Check sheet for the modelled part. Datum: model origin and axes. Units: mm. Face numbers are marked on the shaded views. A direction names the side the tool comes from. Give positions to 0.01 mm unless a question says otherwise; leave off trailing zeros. Order: outer loops, then holes, each group sorted by start corner. A loop starts at its lowest first (then second) coordinate and runs counter-clockwise, first axis right, second up.
Item 1: Gauge pin test, flat ends, axial feed: P1, Ø2, axis at x = 3.5, y = 3.5, coming from the +Z side; P2, Ø9.5, axis at x = 0, z = 0, coming from the -Y side; P3, Ø1.2, axis at x = -4, y = 3.5, coming from the +Z side; P4, Ø1.5, axis at y = 2, z = -35.5, coming from the -X side. Record the tip position at first contact, or that the pin passes through.
Item 2: Sectioned sample at D-D on x = -10. Record the boundary of the cut face in (y, z), and give its area (3 significant figures).
Item 3: Sectioned sample at B-B on z = 0. Record the boundary of the cut face in (x, y), and give its area (3 significant figures).
Item 4: Sectioned sample at A-A on x = 0. Record the boundary of the cut face in (y, z), and give its area (4 significant figures).
Item 5: Release check for a two-part mould opening along X. For the marked faces 3 and 4 record: released by +X, released by -X, zero draft, split by the parting line, or undercut.
Item 6: Access from +Z, -Z, +X, -X, +Y, -Y to the whole of each face (thin tool, end or side, straight path). Record for the marked faces 1 and 2.
Item 7: Material ranges on line 1 along X through (y, z) = (2.15, 0); line 2 along Z through (x, y) = (-3.1, 1.9); line 3 along X through (y, z) = (4.6, 1), recorded low to high.
Item 8: Sectioned sample at C-C on y = 2.6. Record the boundary of the cut face in (x, z), and give its area (3 significant figures).
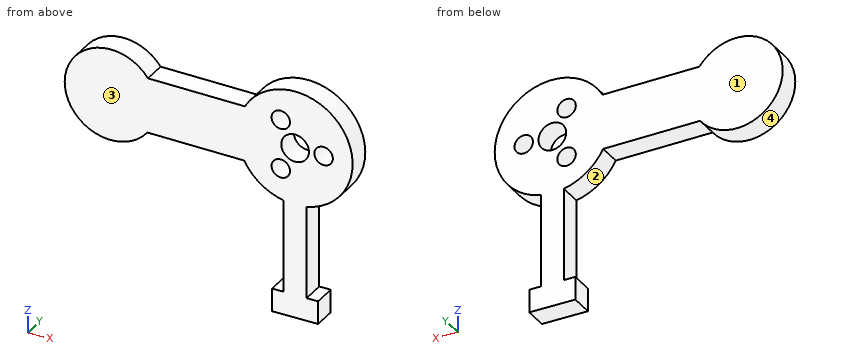
from build123d import *

# Parameters (mm, degrees)
SKETCH1_R           = 2
SKETCH1_R_2         = 3
BOSS_EXTRUDE1_DEPTH = 5


with BuildPart() as part:
    # Sketch1 → Boss-Extrude1 (new body)
    with BuildSketch(Plane(origin=(0, 0, 0), x_dir=(1, 0, 0), z_dir=(0, 1, 0))):
        with BuildLine():
            Line((-31.924309824, -6.390496245), (-10.891735709, -6.133522091))
            ThreePointArc((-10.891735709, -6.133522091), (10.102986142, -7.36068414), (2.5, 12.247448714))
            Line((2.5, 12.247448714), (2.5, 32.4))
            Line((2.5, 32.4), (5, 32.4))
            Line((5, 32.4), (5, 37.4))
            Line((5, 37.4), (-5, 37.4))
            Line((-5, 37.4), (-5, 32.4))
            Line((-5, 32.4), (-2.5, 32.4))
            Line((-2.5, 32.4), (-2.5, 12.247448714))
            ThreePointArc((-2.5, 12.247448714), (-7.483563, 10.012306668), (-11.038339719, 5.865582345))
            Line((-11.038339719, 5.865582345), (-32.070913834, 5.608608191))
            ThreePointArc((-32.070913834, 5.608608191), (-49.996268483, -0.610850042), (-31.924309824, -6.390496245))
        make_face()
        with Locations((6.2, 0)):
            Circle(SKETCH1_R, mode=Mode.SUBTRACT)
        with Locations((-3.1, -5.369357503)):
            Circle(SKETCH1_R, mode=Mode.SUBTRACT)
        Circle(SKETCH1_R_2, mode=Mode.SUBTRACT)
        with Locations((-3.1, 5.369357503)):
            Circle(SKETCH1_R, mode=Mode.SUBTRACT)
    extrude(amount=BOSS_EXTRUDE1_DEPTH)


solid = part.part
Report:
1. P1: stops at z = 12.25
1. P2: stops at y = 0
1. P3: stops at z = 12.03
1. P4: stops at x = -5
2. outline: (0, -7.5) - (5, -7.5) - (5, 7.5) - (0, 7.5) - close
2. area: 75.0 mm2
3. outline: (-49.99, 0) - (-3, 0) - (-3, 5) - (-49.99, 5) - close; (3, 0) - (4.2, 0) - (4.2, 5) - (3, 5) - close; (8.2, 0) - (12.5, 0) - (12.5, 5) - (8.2, 5) - close
3. area: 262 mm2
4. outline: (0, -37.4) - (5, -37.4) - (5, -3) - (0, -3) - close; (0, 3) - (5, 3) - (5, 12.5) - (0, 12.5) - close
4. area: 219.5 mm2
5. face 3: zero draft
5. face 4: undercut
6. face 1: +Z, -Z, +X, -X, +Y
6. face 2: +Y, -Y
7. line 1: x = -49.99 to -3, 3 to 4.2, 8.2 to 12.5
7. line 2: z = -37.4 to -32.4, -12.11 to -7.37, -3.37 to 3.37, 7.37 to 12.11
7. line 3: x = -49.98 to -2.83, 2.83 to 4.47, 7.93 to 12.46
8. outline: (-32.07, -5.61) - (-11.04, -5.87) arc R12.5 ccw to (-2.5, -12.25) - (-2.5, -32.4) - (-5, -32.4) - (-5, -37.4) - (5, -37.4) - (5, -32.4) - (2.5, -32.4) - (2.5, -12.25) arc R12.5 ccw (long way) to (-10.89, 6.13) - (-31.92, 6.39) arc R10 ccw (long way) to start; hole circle Ø4 at (-3.1, -5.37); hole circle Ø4 at (-3.1, 5.37); hole circle Ø6 at (0, 0); hole circle Ø4 at (6.2, 0)
8. area: 1,110 mm2
